Model file for the job. Use its own axes, mm. Face numbers are marked on the shaded views. Round coordinates to 2 decimals unless told otherwise and drop trailing zeros. Order: outer loops, then holes, each group sorted by start corner. A loop starts at its lowest first (then second) coordinate and runs counter-clockwise, first axis right, second up. Notation, with made-up numbers: (-28, 21) -> (-4, 21) arc R7 cw to (-4, 31) -> close; hole circle Ø6 at (61, -31.75). An arc over 180 degrees is marked (long way). Put each result on its own line as item: value. Start each with the question number.
Q1. Flat gauge pins, fed straight in: P1, Ø3, axis at y = 12, z = 58.5, coming from the -X side; P2, Ø1.7, axis at x = 8.5, z = 48.5, coming from the -Y side; P3, Ø2, axis at x = 17.5, z = 31.5, coming from the +Y side; P4, Ø1.5, axis at x = 20, y = 28.5, coming from the +Z side. Where does each tip first touch, or does it go through?
Q2. Cut at A-A, the plane y = 20. List the corners of the cut face in (x, z).
Q3. Cut at C-C, the plane y = 10.25. List the corners of the cut face in (x, z).
Q4. Cut at D-D, the plane z = 7. List the corners of the cut face in (x, y), and give its area (3 significant figures).
Q5. Pull direction X, two halves, no side cores. Call the marked faces 1 and 2: released by +X, released by -X, zero draft, split by the parting line, or undercut.
Q6. Probe L1, parallel to Y at x = 20, z = 30; L2, parallel to X at y = 20, z = 46. List the from-to ranges inside material, lowest first.
Q7. Cut at B-B, the plane x = 14. List the corners of the cut face in (y, z).
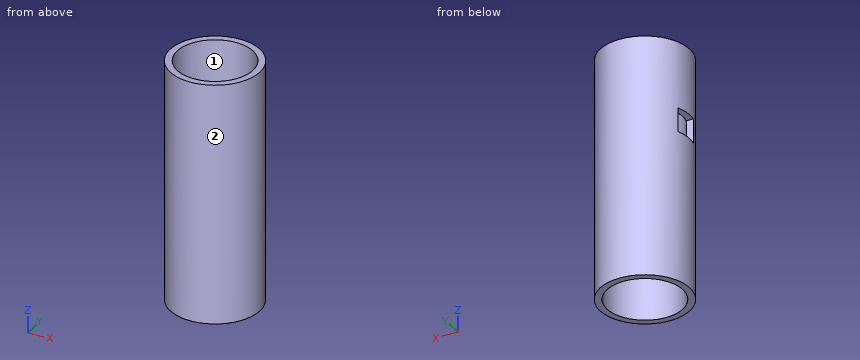
Autodesk Fusion 360 part; units mm, degrees
sketch "Sketch1" plane through (0, 0, 0) normal (0, 0, 1) x (1, 0, 0)
  circle A0 centre (20, 20) radius 13
  dimension "d1" = 26
extrude "Extrude1" add sketch "Sketch1" along normal blind 70
sketch "Sketch2" plane through (0, 0, 70) normal (0, 0, 1) x (1, 0, 0)
  circle A0 centre (20, 20) radius 13
  circle A1 centre (20, 20) radius 11
  dimension "d4" = 2
extrude "Extrude2" cut sketch "Sketch2" against normal up to surface (70 mm away) contours A1
sketch "Sketch3" plane through (0, 0, 0) normal (1, 0, 0) x (0, 0, -1)
  line L0 (-50.7051, 17.6488) -> (-43.7051, 17.6488)
  line L1 (-43.7051, 17.6488) -> (-43.7051, 24.6488)
  line L2 (-43.7051, 24.6488) -> (-50.7051, 24.6488)
  line L3 (-50.7051, 24.6488) -> (-50.7051, 17.6488)
  line L4 (-50.7051, 17.6488) -> (-43.7051, 24.6488) construction
  line L5 (-43.7051, 17.6488) -> (-50.7051, 24.6488) construction
  point P0 (-47.2051, 21.1488)
  dimension "d7" = 7
  dimension "d8" = 7
extrude "Extrude4" cut sketch "Sketch3" along normal blind 15
extrude "Extrude3" cut sketch "Sketch3" along normal blind 12
Ans:
1. P1: stops at x = 8.74
1. P2: stops at y = 12.54
1. P3: stops at y = 32.91
1. P4: passes through
2. outline: (7, 0) -> (9, 0) -> (9, 43.71) -> (7, 43.71) -> close; (7, 50.71) -> (9, 50.71) -> (9, 70) -> (7, 70) -> close; (31, 0) -> (33, 0) -> (33, 70) -> (31, 70) -> close
3. outline: (11.4, 0) -> (14.91, 0) -> (14.91, 70) -> (11.4, 70) -> close; (25.09, 0) -> (28.6, 0) -> (28.6, 70) -> (25.09, 70) -> close
4. outline: circle Ø26 at (20, 20); hole circle Ø22 at (20, 20)
4. area: 151 mm^2
5. face 1: undercut
5. face 2: split by the parting line
6. L1: y = 7 to 9, 31 to 33
6. L2: x = 31 to 33
7. outline: (8.47, 0) -> (10.78, 0) -> (10.78, 70) -> (8.47, 70) -> close; (29.22, 0) -> (31.53, 0) -> (31.53, 70) -> (29.22, 70) -> close
